```python
from build123d import *

# Parameters (mm, degrees)
BOSS_EXTRUDE1_DEPTH = 5
CUT_EXTRUDE3_DEPTH  = 3
FILLET1_R           = 5
FILLET2_R           = 10
FILLET3_R           = 5
FILLET4_R           = 2


with BuildPart() as part:
    # Sketch1 → Boss-Extrude1 (new body)
    with BuildSketch(Plane(origin=(0, 0, 0), x_dir=(1, 0, 0), z_dir=(0, 1, 0))):
        Polygon((0, 5.8), (20, 5.8), (20, 74.2), (31.6, 74.2), (31.6, 5.8), (31.6, -5.8), (20, -5.8), (0, -5.8), (-11.6, -5.8), (-11.6, 29.2), (0, 29.2), align=None)
    extrude(amount=BOSS_EXTRUDE1_DEPTH)

    # Sketch2 → Cut-Extrude3 (cut)
    with BuildSketch(Plane(origin=(0, 5, 0), x_dir=(1, 0, 0), z_dir=(0, 1, 0))):
        with BuildLine():
            Line((28.721, 64.841739258), (27.723587356, 52.636800493))
            ThreePointArc((27.723587356, 52.636800493), (25.8, 50.864), (23.876412644, 52.636800493))
            Line((23.876412644, 52.636800493), (22.879, 64.841739258))
            ThreePointArc((22.879, 64.841739258), (25.8, 70.6), (28.721, 64.841739258))
        make_face()
    extrude(amount=-CUT_EXTRUDE3_DEPTH, mode=Mode.SUBTRACT)

    # Fillet1
    fillet1_edges = [part.edges().sort_by_distance(p)[0] for p in [
        (20, 2.5, -74.2),
        (31.6, 2.5, -74.2),
    ]]
    fillet(fillet1_edges, radius=FILLET1_R)

    # Fillet2
    fillet2_edges = [part.edges().sort_by_distance(p)[0] for p in [
        (31.6, 2.5, 5.8),
        (-11.6, 2.5, 5.8),
    ]]
    fillet(fillet2_edges, radius=FILLET2_R)

    # Fillet3
    fillet3_edges = [part.edges().sort_by_distance(p)[0] for p in [
        (-11.6, 2.5, -29.2),
        (0, 2.5, -29.2),
    ]]
    fillet(fillet3_edges, radius=FILLET3_R)

    # Fillet4
    fillet4_edges = [part.edges().sort_by_distance(p)[0] for p in [
        (0, 2.5, -5.8),
        (20, 2.5, -5.8),
    ]]
    fillet(fillet4_edges, radius=FILLET4_R)


solid = part.part
```
Check sheet for the modelled part. Datum: model origin and axes. Units: mm. A direction names the side the tool comes from. Give positions to 0.01 mm unless a question says otherwise; leave off trailing zeros. Write each loop counter-clockwise with the first axis right and the second up, starting at its lowest first coordinate (ties: lowest second). Pieces come first, ordered by that corner, then holes.
Item 1: Cross-section at B-B (y = 1). Enter the section's corners in (x, z), and give its area (3 significant figures).
Item 2: Gauge pin test, flat ends, axial feed: pin 1 (2 mm diameter, centred on y = 2.5, z = -56.5, fed in from -X); pin 2 (8 mm diameter, centred on x = 25.5, z = -64, fed in from +Y); pin 3 (0.8 mm diameter, centred on x = -5.5, y = 1.5, fed in from -Z); pin 4 (2.5 mm diameter, centred on y = 3, z = -28, fed in from -X). Record the tip position at first contact, or that the pin passes through.
Item 3: Draft check along X on faces 1 (the face through (-10.17, 2.54, -27.7)), 2 (the face through (0.57, 2.54, -6.4)), 3 (the face through (26, 2, -74.2)). Enter one of: released by +X, released by -X, zero draft, split by the parting line, or undercut.
Item 4: Access from +Z, -Z, +X, -X, +Y, -Y to the whole of each face (thin tool, end or side, straight path). Record for faces 4 (the face through (21.43, 2.54, -72.7)), 5 (the face through (25.84, 3.521, -50.864)), 6 (the face through (10, 2, -5.8)).
Item 5: Cross-section at A-A (z = -17). Enter the section's corners in (x, y), and give its area (3 significant figures).
Item 6: Cross-section at D-D (x = 25.8). Enter the section's corners in (y, z), and give its area (3 significant figures).
Item 7: Cross-section at C-C (z = -66.98). Enter the section's corners in (x, y), and give its area (3 significant figures).
Item 8: Scan lines: L1, parallel to X at y = 2.5, z = -13.5; L2, parallel to X at y = 2.6, z = -66.98; L3, parallel to Z at x = 2, y = 4.6. Record each from-to range of solid material in increasing order.
Report:
1. outline: (-11.6, -24.2) arc R5 ccw to (-6.6, -29.2) - (-5, -29.2) arc R5 ccw to (0, -24.2) - (0, -7.8) arc R2 cw to (2, -5.8) - (18, -5.8) arc R2 cw to (20, -7.8) - (20, -69.2) arc R5 ccw to (25, -74.2) - (26.6, -74.2) arc R5 ccw to (31.6, -69.2) - (31.6, -4.2) arc R10 ccw to (21.6, 5.8) - (-1.6, 5.8) arc R10 ccw to (-11.6, -4.2) - close
1. area: 1,500 mm2
2. pin 1: stops at x = 20
2. pin 2: stops at y = 5
2. pin 3: stops at z = -29.2
2. pin 4: stops at x = -10.9
3. face 1: released by -X
3. face 2: undercut
3. face 3: zero draft
4. face 4: -Z, -X, +Y, -Y
4. face 5: +Y
4. face 6: -Z, +Y, -Y
5. outline: (-11.6, 0) - (0, 0) - (0, 5) - (-11.6, 5) - close; (20, 0) - (31.6, 0) - (31.6, 5) - (20, 5) - close
5. area: 116 mm2
6. outline: (0, -74.2) - (5, -74.2) - (5, -70.6) - (2, -70.6) - (2, -50.86) - (5, -50.86) - (5, 4.88) - (0, 4.88) - close
6. area: 336 mm2
7. outline: (20, 0) - (31.6, 0) - (31.6, 5) - (29.42, 5) - (29.42, 2) - (22.18, 2) - (22.18, 5) - (20, 5) - close
7. area: 36.3 mm2
8. L1: x = -11.6 to 0, 20 to 31.6
8. L2: x = 20 to 22.18, 29.42 to 31.6
8. L3: z = -5.8 to 5.8
